Autodesk Inventor part; units mm, degrees
ref_plane "YZ Plane" through (0, 0, 0) normal (1, 0, 0) x (0, 1, 0)
ref_plane "XZ Plane" through (0, 0, 0) normal (0, 1, 0) x (-1, 0, 0)
ref_plane "XY Plane" through (0, 0, 0) normal (0, 0, 1) x (1, 0, 0)
sketch "Sketch1" plane through (0, 0, 0) normal (0, 0, 1) x (1, 0, 0)
  line L0 (-108, 108) -> (108, 108)
  line L1 (108, 108) -> (108, -108)
  line L2 (108, -108) -> (-108, -108)
  line L3 (-108, -108) -> (-108, 108)
  line L4 (-108, 108) -> (108, -108) construction
  line L5 (108, 108) -> (-108, -108) construction
  point P0 (0, 0)
  dimension "d0" = 216
  dimension "d2" = 216
extrude "Extrusion1" add sketch "Sketch1" along normal mid plane 3
sketch "Sketch2" plane through (0, 0, 1.5) normal (0, 0, 1) x (1, 0, 0)
  line L0 (108, 108) -> (-108, 108)
  line L1 (-108, 108) -> (-108, -108)
  line L2 (-108, -108) -> (108, -108)
  line L3 (108, -108) -> (108, 108)
  circle A0 centre (104.5, -104.5) radius 1.8 construction
  line L4 (102.7, -104.5) -> (-104.5, -104.5) construction
  line L5 (104.5, 104.5) -> (-104.5, 104.5) construction
  line L6 (104.5, 104.5) -> (104.5, -104.5) construction
  line L7 (-104.5, 104.5) -> (-104.5, -104.5) construction
  line L8 (0, 104.5) -> (0, -104.5) construction
  point P0 (0, 0)
  point P1 (-102.3056, -104.5)
  point P2 (104.5, 0)
  point P3 (-104.5, 0)
  point P4 (0, 0)
  dimension "d6" = 3.6
  dimension "d5" = 3.5
  dimension "d7" = 1.7
  dimension "d8" = 3.5
  dimension "d9" = 3.5
  dimension "d10" = 3.5
  dimension "d11" = 3.5
  dimension "d13" = 108
hole "Hole1" at (104.5, 104.5, 1.5) at (104.5, -104.5, 1.5) at (-102.3056, -104.5, 1.5) at (-104.5, 104.5, 1.5) at (104.5, 0, 1.5) at (-104.5, 0, 1.5) at (0, 104.5, 1.5) at (0, -104.5, 1.5) at (0, 0, 1.5) direction (0, 0, -1) diameter 3.6 end through all
sketch "Sketch3" plane through (0, 0, 1.5) normal (0, 0, 1) x (1, 0, 0)
  line L0 (108, 108) -> (-108, 108)
  line L1 (-108, 108) -> (-108, -108)
  line L2 (108, -108) -> (108, 108)
  line L3 (-108, 82.65) -> (108, 82.65) construction
  line L4 (-108, 69) -> (108, 69) construction
  point P0 (-52.3, 82.65)
  point P1 (-42.3, 82.65)
  point P2 (-32.3, 82.65)
  point P3 (-22.3, 82.65)
  point P4 (20.32, 69)
  point P5 (30.32, 69)
  point P6 (40.32, 69)
  point P7 (50.32, 69)
  dimension "d21" = 25.35
  dimension "d23" = 39
  dimension "d24" = 160.3
  dimension "d25" = 150.3
  dimension "d26" = 140.3
  dimension "d27" = 130.3
  dimension "d28" = 57.68
  dimension "d29" = 67.68
  dimension "d30" = 77.68
  dimension "d31" = 87.68
hole "Hole2" at (-52.3, 82.65, 1.5) at (-42.3, 82.65, 1.5) at (-32.3, 82.65, 1.5) at (-22.3, 82.65, 1.5) at (20.32, 69, 1.5) at (30.32, 69, 1.5) at (40.32, 69, 1.5) at (50.32, 69, 1.5) direction (0, 0, -1) diameter 7.14 end through all
sketch "Sketch4" plane through (0, 0, 1.5) normal (0, 0, 1) x (1, 0, 0)
  line L0 (-108, 108) -> (-108, -108)
  line L1 (108, -108) -> (108, 108)
  line L2 (-108, 82.65) -> (108, 82.65) construction
  line L3 (-108, 69) -> (108, 69) construction
  point P0 (-50.32, 69)
  point P1 (-40.32, 69)
  point P2 (-30.32, 69)
  point P3 (-20.32, 69)
  point P4 (22.3, 82.65)
  point P5 (32.3, 82.65)
  point P6 (42.3, 82.65)
  point P7 (52.3, 82.65)
  dimension "d125" = 158.32
  dimension "d126" = 148.32
  dimension "d127" = 138.32
  dimension "d128" = 128.32
  dimension "d129" = 55.7
  dimension "d130" = 65.7
  dimension "d131" = 75.7
  dimension "d132" = 85.7
hole "Hole3" at (-50.32, 69, 1.5) at (-40.32, 69, 1.5) at (-30.32, 69, 1.5) at (-20.32, 69, 1.5) at (22.3, 82.65, 1.5) at (32.3, 82.65, 1.5) at (42.3, 82.65, 1.5) at (52.3, 82.65, 1.5) direction (0, 0, -1) diameter 5 end through all
sketch "Sketch5" plane through (0, 0, 1.5) normal (0, 0, 1) x (1, 0, 0)
  circle A0 centre (0, 0) radius 1.8
  line L0 (-108, 108) -> (-108, -108)
  line L1 (108, -108) -> (108, 108)
  line L2 (-108, 55.35) -> (108, 55.35) construction
  point P0 (-32.3, 55.35)
  dimension "d46" = 55.35
  dimension "d47" = 75.7
hole "Hole4" at (-32.3, 55.35, 1.5) direction (0, 0, -1) diameter 5 end through all
sketch "Sketch6" plane through (0, 0, 1.5) normal (0, 0, 1) x (1, 0, 0)
  circle A0 centre (-32.3, 55.35) radius 2.5
  point P0 (32.3, 55.35)
  dimension "d55" = 64.6
hole "Hole5" at (32.3, 55.35, 1.5) direction (0, 0, -1) diameter 7.14 end through all
mirror "Mirror1" about plane through (0, 0, 0) normal (0, 1, 0) of "Hole2", "Hole3", "Hole4", "Hole5"
sketch "Sketch7" plane through (0, 0, 1.5) normal (0, 0, 1) x (1, 0, 0)
  circle A0 centre (0, 0) radius 1.8
  point P0 (-10, 0)
  point P1 (10, 0)
  dimension "d63" = 10
  dimension "d64" = 10
hole "Hole6" at (-10, 0, 1.5) at (10, 0, 1.5) direction (0, 0, -1) diameter 5 end through all
sketch "Sketch8" plane through (0, 0, 1.5) normal (0, 0, 1) x (1, 0, 0)
  line L0 (108, 108) -> (-108, 108)
  line L1 (-108, 108) -> (-108, -108)
  line L2 (108, -108) -> (108, 108)
  line L3 (2.5, 15.2915) -> (2.5, 28) construction
  point P0 (12.64, 15.17)
  point P1 (12.64, 28)
  dimension "d72" = 80
  dimension "d73" = 10.14
  dimension "d74" = 12.83
  dimension "d75" = 110.5
hole "Hole7" at (2.5, 15.2915, 1.5) at (12.64, 15.17, 1.5) at (12.64, 28, 1.5) at (2.5, 28, 1.5) direction (0, 0, -1) diameter 3.5 end through all
sketch "Sketch9" plane through (0, 0, 1.5) normal (0, 0, 1) x (1, 0, 0)
  line L0 (108, 108) -> (-108, 108)
  line L1 (-108, 108) -> (-108, -108)
  point P0 (14, 45)
  point P1 (23.12, 45)
  dimension "d83" = 122
  dimension "d84" = 63
  dimension "d85" = 9.12
hole "Hole8" at (14, 45, 1.5) at (23.12, 45, 1.5) direction (0, 0, -1) diameter 3.14 end through all
sketch "Sketch10" plane through (0, 0, 1.5) normal (0, 0, 1) x (1, 0, 0)
  circle A0 centre (14, 45) radius 1.57
  line L0 (-108, -108) -> (108, -108)
  line L1 (108, -108) -> (108, 108)
  line L2 (14, 45) -> (14, -40) construction
  point P0 (23.12, -40)
  dimension "d93" = 68
  dimension "d94" = 9.12
hole "Hole9" at (14, -40, 1.5) at (23.12, -40, 1.5) direction (0, 0, -1) diameter 3.14 end through all
sketch "Sketch11" plane through (0, 0, 1.5) normal (0, 0, 1) x (1, 0, 0)
  circle A0 centre (0, -104.5) radius 1.8
  line L0 (-108, -108) -> (108, -108)
  line L1 (-3.25, -97.12) -> (3.25, -97.12)
  line L2 (3.25, -97.12) -> (3.25, -100.12)
  line L3 (3.25, -100.12) -> (-3.25, -100.12)
  line L4 (-3.25, -100.12) -> (-3.25, -97.12)
  line L5 (-3.25, -97.12) -> (3.25, -100.12) construction
  line L6 (3.25, -97.12) -> (-3.25, -100.12) construction
  arc A1 (-3.25, -97.12) -> (-3.25, -100.12) centre (-3.25, -98.62) ccw
  arc A2 (3.25, -100.12) -> (3.25, -97.12) centre (3.25, -98.62) ccw
  point P0 (0, -98.62)
  dimension "d104" = 9.38
  dimension "d105" = 6.5
  dimension "d106" = 3
extrude "Extrusion2" cut sketch "Sketch11" against normal through all contours L1 L2 L3 L4 | L4 A1 | A2 L2
sketch "Sketch12" plane through (0, 0, 1.5) normal (0, 0, 1) x (1, 0, 0)
  circle A0 centre (0, -104.5) radius 1.8
  line L0 (-108, -108) -> (108, -108)
  line L1 (-10, -66.5) -> (10, -66.5)
  line L2 (10, -66.5) -> (10, -71.5)
  line L3 (10, -71.5) -> (-10, -71.5)
  line L4 (-10, -71.5) -> (-10, -66.5)
  line L5 (-10, -66.5) -> (10, -71.5) construction
  line L6 (10, -66.5) -> (-10, -71.5) construction
  arc A1 (-10, -66.5) -> (-10, -71.5) centre (-10, -69) ccw
  arc A2 (10, -71.5) -> (10, -66.5) centre (10, -69) ccw
  point P0 (0, -69)
  dimension "d109" = 5
  dimension "d111" = 39
  dimension "d112" = 20
extrude "Extrusion3" cut sketch "Sketch12" against normal through all contours L1 L2 L3 L4 | L4 A1 | A2 L2
mirror "Mirror2" about plane through (0, 0, 0) normal (0, 1, 0) of "Extrusion2", "Extrusion3"
sketch "Sketch13" plane through (0, 0, 1.5) normal (0, 0, 1) x (1, 0, 0)
  circle A0 centre (104.5, 104.5) radius 1.8
  line L0 (108, 108) -> (-108, 108)
  point P0 (83, 102.92)
  point P1 (83, 72)
  dimension "d115" = 1.58
  dimension "d116" = 21.5
  dimension "d117" = 36
hole "Hole10" at (83, 102.92, 1.5) at (83, 72, 1.5) direction (0, 0, -1) diameter 3.6 end through all
fillet "Fillet1" radius 1.75 4 edges at (-108, -108, 0) (-108, 108, 0) (108, -108, 0) (108, 108, 0)
properties part number "V-Slot Universal Build Pate" material "Aluminum 6061"
Design review of the part built by this model. Coordinates are the model's own, in mm. Coordinates: 2 decimals unless noted, no trailing zeros. Loops run counter-clockwise (first coordinate to the right, second up) from the corner with the lowest first, then second, coordinate; pieces in that order, holes last.
Q1. We need section A-A on y = -55.35. State the section outline as (x, z) points.
Reported:
outline: (-108, -1.5) - (-34.8, -1.5) - (-34.8, 1.5) - (-108, 1.5) - close; (-29.8, -1.5) - (28.73, -1.5) - (28.73, 1.5) - (-29.8, 1.5) - close; (35.87, -1.5) - (108, -1.5) - (108, 1.5) - (35.87, 1.5) - close
Q2. We need section B-B on z = 0.15. State how many separate pieces and enclosed holes the cut face has, and give its area (3 significant figures).
Reported:
separate pieces: 1
enclosed holes: 61
area: 45,100 mm2
Q3. To check wall thickness, follow line 1 (Y direction, x = -10, z = 0.3); line 2 (X direction, y = 28, z = 0); line 3 (X direction, y = 0, z = 0.55). State the ranges of each line that lie inside material, in increasing order.
Reported:
line 1: y = -108 to -71.5, -66.5 to -2.5, 2.5 to 66.5, 71.5 to 108
line 2: x = -108 to 0.75, 4.25 to 10.89, 14.39 to 108
line 3: x = -108 to -106.3, -102.7 to -12.5, -7.5 to -1.8, 1.8 to 7.5, 12.5 to 102.7, 106.3 to 108
Q4. The part is to be moulded in two halves that separate along X. For faces 1 (the face through (30.933, -52.052, -0.021)), 2 (the face through (-45.467, -81.003, -0.021)), 3 (the face through (-2, 2, -1.5)), say which applies: +X half, -X half, draft (parallel to the pull), parting line (faces both ways), or undercut.
Reported:
face 1: undercut
face 2: undercut
face 3: draft
Q5. For pin 1 (4.5 mm diameter, centred on x = 20.32, y = -69, fed in from -Z), flat-tipped, find the tip position at first contact; note if it passes through.
Reported:
pin 1: passes through
